For this review, use the dimensioned drawing (mm, ordinates from the lowest corner) and the shaded views. A direction names the side the tool comes from. Give positions to 0.01 mm unless a question says otherwise; leave off trailing zeros. Order: outer loops, then holes, each group sorted by start corner. A loop starts at its lowest first (then second) coordinate and runs counter-clockwise, first axis right, second up. Notation, with made-up numbers: M 66,42 L 119,42 A9 cw 119,48 Z; hole C 85.25,84.5 d11. An arc over 180 degrees is marked long. Use CSV: the item, a comma, the result in double quotes. Start each with the question number.
(1) Clearance check with flat-ended pins moving along their axes: P1, Ø8, axis at x = 4.5, z = 18.5, coming from the +Y side; P2, Ø5, axis at x = 21.5, z = 4.5, coming from the +Y side (3 decimals); P3, Ø6, axis at x = 13, z = 5.5, coming from the +Y side. State where each tip first meets the part, or that it passes through.
(2) Wall thickness on L1, parallel to Z at x = 23.5, y = 12.5; L2, parallel to Y at x = 3, z = 14; L3, parallel to Y at x = 20.25, z = 14.5: over which ranges is each line inside the solid? List them lowest first. Write a range as from..to.
(3) Consider section A-A (y = 12.5). Write out the cut boundary in (x, z), and give its area (3 significant figures).
(4) Consider section D-D (x = 14.5). Write out the cut boundary in (y, z).
(5) Draft analysis for pull direction Z (two halves, no side actions). For the marked faces 3, 4 and 5, state which applies: pulls with the +Z half, pulls with the -Z half, needs draft (parallel to the pull), parting line crosses it, or undercut.
(6) Consider section C-C (x = 20.5). Write out the cut boundary in (y, z).
(7) Tool access review of the marked faces 1 and 2: name each direction out of +Z, -Z, +X, -X, +Y, -Y from which nothing blocks a thin tool from reaching the whole face with its end or side.
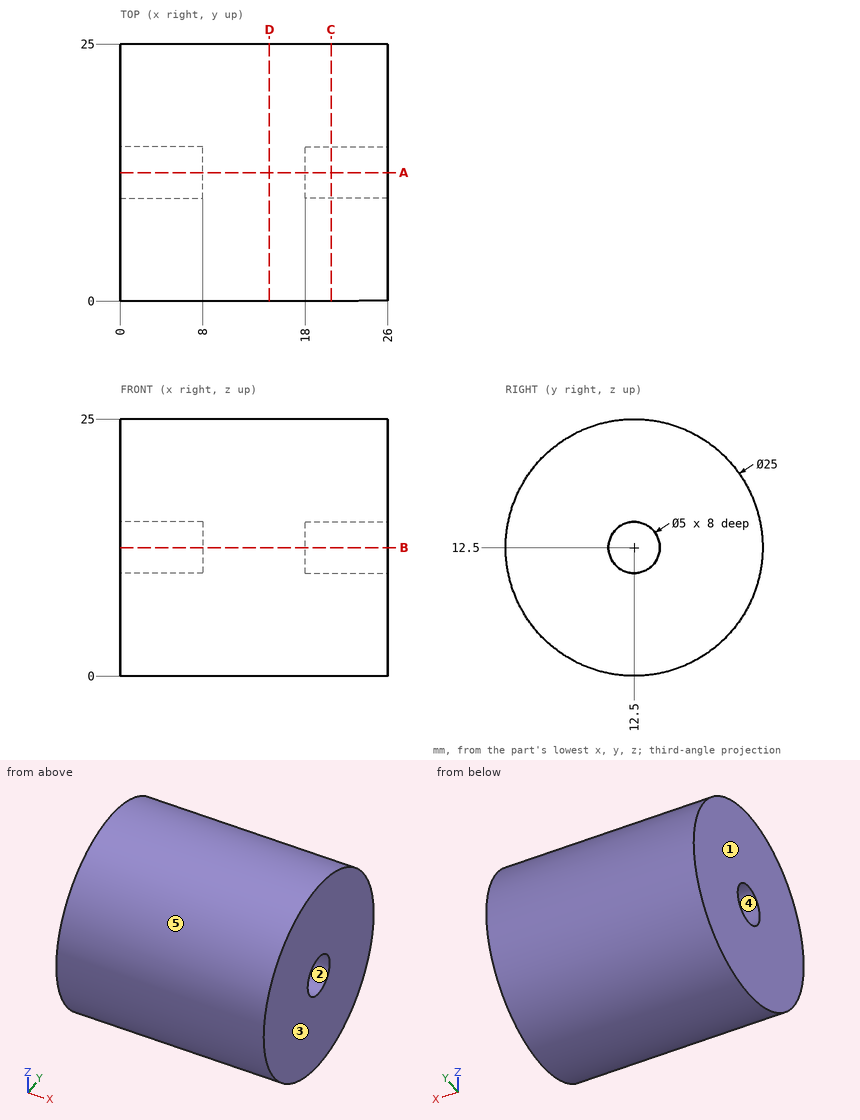
Check result:
1,P1,"stops at y = 24.84"
1,P2,"stops at y = 23.725"
1,P3,"stops at y = 24.34"
2,L1,"z = 0..10, 15..25"
2,L2,"y = 0.09..10.5, 14.5..24.91"
2,L3,"y = 0.16..11, 14..24.84"
3,outline,"M 0,0 L 26,0 L 26,10 L 18,10 L 18,15 L 26,15 L 26,25 L 0,25 L 0,15 L 8,15 L 8,10 L 0,10 Z"
3,area,"570 mm^2"
4,outline,"C 12.5,12.5 d25"
5,face 3,"needs draft"
5,face 4,"undercut"
5,face 5,"parting line crosses it"
6,outline,"C 12.5,12.5 d25; hole C 12.5,12.5 d5"
7,face 1,"+Z, -Z, -X, +Y, -Y"
7,face 2,"+X"
